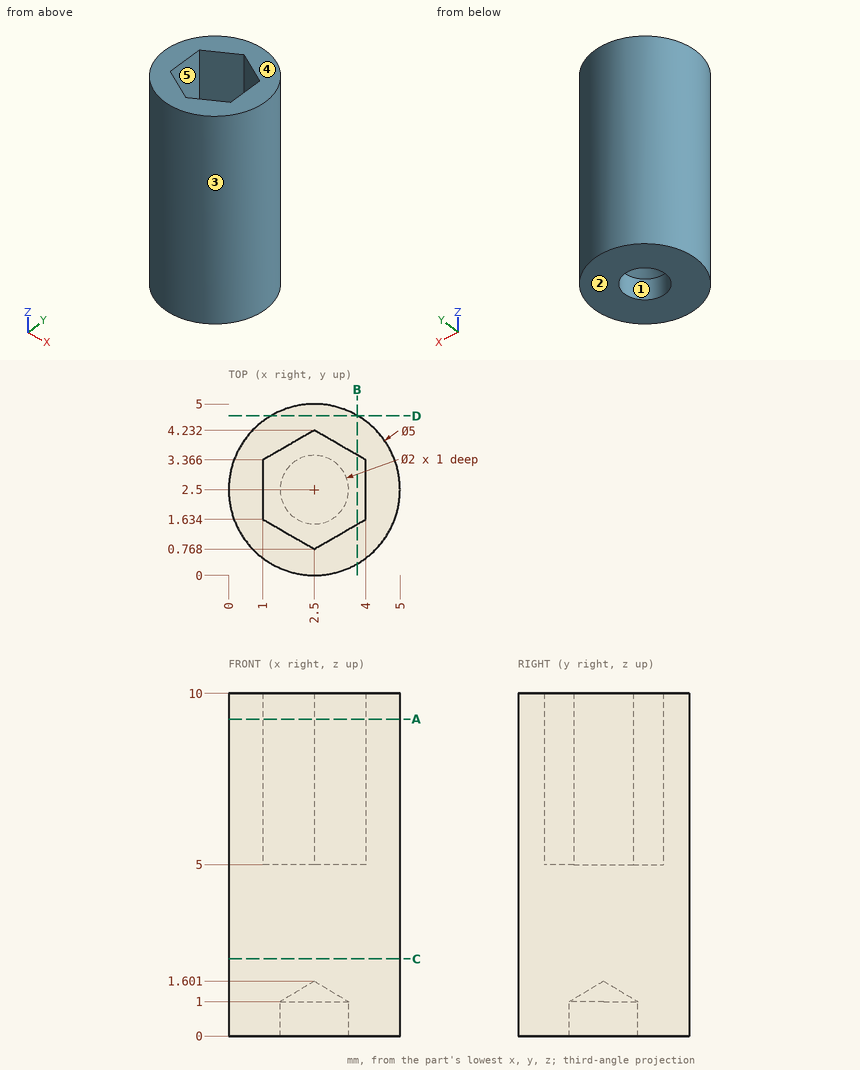
Job drawing, mm, ordinate dimensions from the low corner. One solid piece. A direction names the side the tool comes from. Round coordinates to 2 decimals unless told otherwise and drop trailing zeros. Loops run counter-clockwise (first coordinate to the right, second up) from the corner with the lowest first, then second, coordinate; pieces in that order, holes last. Notation, with made-up numbers: (69, -11) -> (76, -11) arc R32 ccw to (76, 18) -> close; hole circle Ø6 at (52.5, 43). An arc over 180 degrees is marked (long way). One line per item, written item: value. Start each with the question number.
Q1. Cut at D-D on y = 4.65. List the corners of the cut face in (x, z), plus the area to 3 significant figures.
Q2. Two-plate mould, pull along Y, no slides. Class the marked faces 1, 2 and 3: released by +Y, released by -Y, zero draft, split by the parting line, or undercut.
Q3. Probe line 1 along Y through (x, z) = (2.5, 0.5); line 2 along Z through (x, y) = (1.5, 1.65); line 3 along X through (y, z) = (3.25, 5.5) (1 decimal). List the from-to ranges inside material, lowest first.
Q4. Cut at A-A on z = 9.25. List the corners of the cut face in (x, y).
Q5. Cut at C-C on z = 2.25. List the corners of the cut face in (x, y), plus the area to 3 significant figures.
Q6. Drop flat-ended pins along their axis: pin 1 Ø1.5 at (x, y) = (3, 2.5) entering from +Z; pin 2 Ø1 at (y, z) = (0.5, 6) entering from +X; pin 3 Ø1.8 at (x, y) = (2.5, 2.5) entering from -Z. Give the stop position or say it passes through.
Q7. Cut at B-B on x = 3.75. List the corners of the cut face in (y, z) (1 decimal).
Q8. 3-axis set-ups, long thin cutter, end or side, ignore diameter. For the marked faces 4 and 5: which of +Z, -Z, +X, -X, +Y, -Y reach the whole face in a straight line?
Computed:
1. outline: (1.22, 0) -> (3.78, 0) -> (3.78, 10) -> (1.22, 10) -> close
1. area: 25.5 mm²
2. face 1: undercut
2. face 2: zero draft
2. face 3: split by the parting line
3. line 1: 0 to 1.5, 3.5 to 5
3. line 2: 0 to 5
3. line 3: 0.1 to 1, 4 to 4.9
4. outline: circle Ø5 at (2.5, 2.5); hole (1, 1.63) -> (2.5, 0.77) -> (4, 1.63) -> (4, 3.37) -> (2.5, 4.23) -> (1, 3.37) -> close
5. outline: circle Ø5 at (2.5, 2.5)
5. area: 19.6 mm²
6. pin 1: z = 5
6. pin 2: x = 4.5
6. pin 3: z = 1.06
7. outline: (0.3, 0) -> (4.7, 0) -> (4.7, 10) -> (3.5, 10) -> (3.5, 5) -> (1.5, 5) -> (1.5, 10) -> (0.3, 10) -> close
8. face 4: +Z, +X, -X, +Y, -Y
8. face 5: +Z
